from build123d import *

# Parameters (mm, degrees)
EXTRUDE_1_DEPTH             = 3
FILLET_1_R                  = 5
SKETCH_2_R                  = 1.5
CUT_EXTRUDE_1_DEPTH         = 113.539992891
SKETCH_4_R                  = 1.5
CUT_EXTRUDE_2_DEPTH         = 113.539992891
SKETCH_6_R                  = 1.5
CUT_EXTRUDE_3_DEPTH         = 113.539992891
SKETCH_7_W                  = 81
SKETCH_7_H                  = 32
CUT_EXTRUDE_4_DEPTH         = 113.539992891
FILLET_2_R                  = 10
SKETCH_8_W                  = 36
SKETCH_8_H                  = 14
CUT_EXTRUDE_5_DEPTH         = 113.539992891
FILLET_3_R                  = 2
HOLE_WIZARD_M3_1_AT_2_COUNT = 2
HOLE_WIZARD_M3_1_AT_2_PITCH = 25
HOLE_WIZARD_M3_1_AT_3_COUNT = 2
HOLE_WIZARD_M3_1_AT_3_PITCH = 65
HOLE_WIZARD_M3_1_AT_4_COUNT = 2
HOLE_WIZARD_M3_1_AT_4_PITCH = 90


with BuildPart() as part:
    # 草图1 → 凸台-拉伸1 (new body)
    with BuildSketch(Plane.XY):
        Polygon((51.5, 90), (-51.5, 90), (-51.5, 70), (-67.5, 70), (-67.5, 32), (-51.5, 32), (-51.5, 0), (51.5, 0), (51.5, 32), (67.5, 32), (67.5, 70), (51.5, 70), align=None)
    extrude(amount=EXTRUDE_1_DEPTH)

    # 圆角1
    fillet_1_edges = [part.edges().sort_by_distance(p)[0] for p in [
        (-51.5, 70, 1.5),
        (-51.5, 90, 1.5),
        (51.5, 90, 1.5),
        (51.5, 70, 1.5),
        (67.5, 70, 1.5),
        (67.5, 32, 1.5),
        (51.5, 32, 1.5),
        (-51.5, 32, 1.5),
        (-67.5, 32, 1.5),
        (-67.5, 70, 1.5),
    ]]
    fillet(fillet_1_edges, radius=FILLET_1_R)

    # 草图2 → 切除-拉伸1 (cut, through all)
    with BuildSketch(Plane.XY.offset(3)):
        with Locations((-45, 82.5)):
            Circle(SKETCH_2_R)
        with Locations(Location((45, 82.5, 0), (0, 0, 180))):
            Circle(SKETCH_2_R)
        with Locations((-20, 82.5)):
            Circle(SKETCH_2_R)
        with Locations(Location((20, 82.5, 0), (0, 0, 180))):
            Circle(SKETCH_2_R)
        with Locations((-60, 60)):
            Circle(SKETCH_2_R)
        with Locations(Location((60, 60, 0), (0, 0, 180))):
            Circle(SKETCH_2_R)
        with Locations((-60, 40)):
            Circle(SKETCH_2_R)
        with Locations(Location((60, 40, 0), (0, 0, 180))):
            Circle(SKETCH_2_R)
    extrude(amount=-CUT_EXTRUDE_1_DEPTH, mode=Mode.SUBTRACT)

    # 草图4 → 切除-拉伸2 (cut, through all)
    with BuildSketch(Plane.XY.offset(3)):
        with Locations((-46.5, 34.5)):
            Circle(SKETCH_4_R)
        with Locations((-23.5, 34.5)):
            Circle(SKETCH_4_R)
        with Locations((-23.5, 8.5)):
            Circle(SKETCH_4_R)
        with Locations((-46.5, 8.5)):
            Circle(SKETCH_4_R)
        with Locations(Location((46.5, 8.5, 0), (0, 0, 180))):
            Circle(SKETCH_4_R)
        with Locations(Location((23.5, 8.5, 0), (0, 0, 180))):
            Circle(SKETCH_4_R)
        with Locations(Location((23.5, 34.5, 0), (0, 0, 180))):
            Circle(SKETCH_4_R)
        with Locations(Location((46.5, 34.5, 0), (0, 0, 180))):
            Circle(SKETCH_4_R)
    extrude(amount=-CUT_EXTRUDE_2_DEPTH, mode=Mode.SUBTRACT)

    # 草图6 → 切除-拉伸3 (cut, through all)
    with BuildSketch(Plane.XY.offset(3)):
        with Locations((0, 19.5)):
            Circle(SKETCH_6_R)
    extrude(amount=-CUT_EXTRUDE_3_DEPTH, mode=Mode.SUBTRACT)

    # 草图7 → 切除-拉伸4 (cut, through all)
    with BuildSketch(Plane.XY.offset(3)):
        with Locations((0, 54)):
            Rectangle(SKETCH_7_W, SKETCH_7_H)
    extrude(amount=-CUT_EXTRUDE_4_DEPTH, mode=Mode.SUBTRACT)

    # 圆角2
    fillet_2_edges = [part.edges().sort_by_distance(p)[0] for p in [
        (40.5, 70, 1.5),
        (40.5, 38, 1.5),
        (-40.5, 38, 1.5),
        (-40.5, 70, 1.5),
    ]]
    fillet(fillet_2_edges, radius=FILLET_2_R)

    # 草图8 → 切除-拉伸5 (cut, through all)
    with BuildSketch(Plane.XY.offset(3)):
        with Locations((0, 31)):
            Rectangle(SKETCH_8_W, SKETCH_8_H)
    extrude(amount=-CUT_EXTRUDE_5_DEPTH, mode=Mode.SUBTRACT)

    # 圆角3
    fillet_3_edges = [part.edges().sort_by_distance(p)[0] for p in [
        (-18, 24, 1.5),
        (-18, 38, 1.5),
        (18, 38, 1.5),
        (18, 24, 1.5),
    ]]
    fillet(fillet_3_edges, radius=FILLET_3_R)

    # 草图9 → M3 六角凹锥坑螺钉的锥形沉头孔1 (revolve, cut)
    with BuildSketch(Plane(origin=(-45, 82.5, 3), x_dir=(0, -1, 0), z_dir=(1, 0, 0))):
        Polygon((0, 0), (0, 3), (1.7, 3), (1.7, 1.66), (3.36, 0), align=None)
    hole_wizard_m3_1 = revolve(axis=Axis((-45, 82.5, 9.35), (0, 0, -1)), mode=Mode.SUBTRACT)

    # M3 六角凹锥坑螺钉的锥形沉头孔1 at 2: M3 六角凹锥坑螺钉的锥形沉头孔1 ×2
    with Locations(*[(i * HOLE_WIZARD_M3_1_AT_2_PITCH, 0, 0) for i in range(1, HOLE_WIZARD_M3_1_AT_2_COUNT)]):
        add(hole_wizard_m3_1, mode=Mode.SUBTRACT)

    # M3 六角凹锥坑螺钉的锥形沉头孔1 at 3: M3 六角凹锥坑螺钉的锥形沉头孔1 ×2
    with Locations(*[(i * HOLE_WIZARD_M3_1_AT_3_PITCH, 0, 0) for i in range(1, HOLE_WIZARD_M3_1_AT_3_COUNT)]):
        add(hole_wizard_m3_1, mode=Mode.SUBTRACT)

    # M3 六角凹锥坑螺钉的锥形沉头孔1 at 4: M3 六角凹锥坑螺钉的锥形沉头孔1 ×2
    with Locations(*[(i * HOLE_WIZARD_M3_1_AT_4_PITCH, 0, 0) for i in range(1, HOLE_WIZARD_M3_1_AT_4_COUNT)]):
        add(hole_wizard_m3_1, mode=Mode.SUBTRACT)


solid = part.part
Geometry: final body of the model. Coordinates: model frame, mm. A direction names the side the tool comes from. Give positions to 0.01 mm unless a question says otherwise; leave off trailing zeros. Write each loop counter-clockwise with the first axis right and the second up, starting at its lowest first coordinate (ties: lowest second). Pieces come first, ordered by that corner, then holes. Notation, with made-up numbers: (-17.5, 43) - (18.5, 43) arc R32 ccw to (18.5, 77) - close; hole circle Ø5 at (4, -22.5). An arc over 180 degrees is marked (long way). Return JSON: item names as keys, results as strings. Group by question number.
1) Section D-D on y = 82.5. Return the cut outline in (x, z), plus the area to 3 significant figures.
2) Mould query, pull axis Y, two halves, no side actions, for faces 5 (the cylindrical face through (66, 33.43, 1.52)), 6 (the cylindrical face through (-37.49, 40.85, 1.48)), 7 (the flat face through (51.5, 80, 1)). Classes: released by +Y, released by -Y, zero draft, split by the parting line, or undercut.
3) Section B-B on x = 7. Return the cut outline in (y, z), plus the area to 3 significant figures.
4) First-contact query: P1, Ø5, axis at x = -45.5, y = 57, coming from the -Z side; P2, Ø1.5, axis at y = 81.5, z = 1, coming from the +X side; P3, Ø1.5, axis at y = 29.5, z = 1.5, coming from the +X side. Flat tips, straight axial feed; report the tip coordinate or a pass-through.
5) Set-up query: faces 1 (the flat face through (-40.5, 54, 2)), 2 (the flat face through (-51.5, 14, 1)), 3 (the flat face through (51.5, 13, 1)), 4 (the cylindrical face through (-50, 88.57, 1.52)). Return all of +Z, -Z, +X, -X, +Y, -Y with unobstructed straight access to the full face (end or side cutting, diameter ignored); none if empty.
6) Line query: line 1 (X direction, y = 49, z = 0.55); line 2 (Y direction, x = 60, z = 2.15); line 3 (Y direction, x = -7, z = 2.6). Output: solid intervals per line, ascending.
7) Section C-C on x = 60. Return the cut outline in (y, z), plus the area to 3 significant figures.
8) Section A-A on y = 8.5. Return the cut outline in (x, z), plus the area to 3 significant figures.
Filled in:
{
 "1": {"outline": "(-51.5, 0) - (-46.7, 0) - (-46.7, 1.34) - (-48.36, 3) - (-51.5, 3) - close; (-43.3, 0) - (-21.7, 0) - (-21.7, 1.34) - (-23.36, 3) - (-41.64, 3) - (-43.3, 1.34) - close; (-18.3, 0) - (18.3, 0) - (18.3, 1.34) - (16.64, 3) - (-16.64, 3) - (-18.3, 1.34) - close; (21.7, 0) - (43.3, 0) - (43.3, 1.34) - (41.64, 3) - (23.36, 3) - (21.7, 1.34) - close; (46.7, 0) - (51.5, 0) - (51.5, 3) - (48.36, 3) - (46.7, 1.34) - close", "area": "257 mm^2"},
 "2": {"face 5": "released by -Y", "face 6": "undercut", "face 7": "zero draft"},
 "3": {"outline": "(0, 0) - (24, 0) - (24, 3) - (0, 3) - close; (70, 0) - (90, 0) - (90, 3) - (70, 3) - close", "area": "132 mm^2"},
 "4": {"P1": "stops at z = 0", "P2": "stops at x = 51.5", "P3": "stops at x = 52.7"},
 "5": {"face 1": "+Z, -Z", "face 2": "+Z, -Z, -X, -Y", "face 3": "+Z, -Z, +X, -Y", "face 4": "+Z, -Z, -X, +Y"},
 "6": {"line 1": "x = -67.5 to -40.5, 40.5 to 67.5", "line 2": "y = 32 to 38.5, 41.5 to 58.5, 61.5 to 70", "line 3": "y = 0 to 24, 70 to 90"},
 "7": {"outline": "(32, 0) - (38.5, 0) - (38.5, 3) - (32, 3) - close; (41.5, 0) - (58.5, 0) - (58.5, 3) - (41.5, 3) - close; (61.5, 0) - (70, 0) - (70, 3) - (61.5, 3) - close", "area": "96.0 mm^2"},
 "8": {"outline": "(-51.5, 0) - (-48, 0) - (-48, 3) - (-51.5, 3) - close; (-45, 0) - (-25, 0) - (-25, 3) - (-45, 3) - close; (-22, 0) - (22, 0) - (22, 3) - (-22, 3) - close; (25, 0) - (45, 0) - (45, 3) - (25, 3) - close; (48, 0) - (51.5, 0) - (51.5, 3) - (48, 3) - close", "area": "273 mm^2"}
}
